Can you work these out from the model? Positions are in its coordinate system, mm. Round coordinates to 2 decimals unless told otherwise and drop trailing zeros.
Q1. Please list where these lines run through material, in increasing order: line 1 along Y through (x, z) = (-75, 12.5); line 2 along Y through (x, z) = (0, 32); line 3 along X through (y, z) = (46.5, 26).
Q2. We'd pull the mould along Y, two halves only. Please class faces 1 (the cylindrical face through (-19.527, 148.724, 39.44)), 2 (the cylindrical face through (-4.357, 54.908, 39.44)), 3 (the flat face through (32, -1, 80)), 4 (the cylindrical face through (23.1, 125.81, 39.44)): +Y half, -Y half, draft (parallel to the pull), parting line (faces both ways), or undercut.
Q3. If we section it at A-A (y = 0): Give the number of separate pieces and of enclosed holes in the cut face, plus the area to 3 significant figures.
Q4. I'm going to push flat-ended pins straight in: pin 1 Ø2 at (y, z) = (-83, 17.5) entering from -X; pin 2 Ø1.5 at (y, z) = (12.5, 24.5) entering from +X; pin 3 Ø8 at (y, z) = (17, 11.5) entering from +X. Where does each tip first touch, or does it pass through?
from build123d import *

# Parameters (mm, degrees)
SKETCH1_R           = 150
BOSS_EXTRUDE1_DEPTH = 80
BOSS_EXTRUDE2_DEPTH = 80
LOFT1_DEPTH         = 80
CIRPATTERN1_COUNT   = 5
FILLET1_R           = 20
FILLET2_R           = 20
FILLET3_R           = 20
SKETCH3_R           = 25
CUT_EXTRUDE1_DEPTH  = 80


with BuildPart() as part:
    # Sketch1 → Boss-Extrude1 (new body)
    with BuildSketch(Plane.XY):
        Circle(SKETCH1_R)
        with BuildLine():
            Line((129.710171657, 8.675907367), (119.956691368, 8.625091073))
            Line((119.956691368, 8.625091073), (120.040051321, -7.374691773))
            Line((120.040051321, -7.374691773), (129.793531611, -7.323875479))
            ThreePointArc((129.793531611, -7.323875479), (105.568888587, -75.86309882), (48.333925621, -120.680701166))
            Line((48.333925621, -120.680701166), (45.271605291, -111.420293279))
            Line((45.271605291, -111.420293279), (30.080667198, -116.443778112))
            Line((30.080667198, -116.443778112), (33.142987529, -125.704185999))
            ThreePointArc((33.142987529, -125.704185999), (-39.527513828, -123.84496619), (-99.838162814, -83.260682474))
            Line((-99.838162814, -83.260682474), (-91.977300573, -77.486619356))
            Line((-91.977300573, -77.486619356), (-101.449176589, -64.591520879))
            Line((-101.449176589, -64.591520879), (-109.310038829, -70.365583996))
            ThreePointArc((-109.310038829, -70.365583996), (-129.998235624, -0.677299621), (-110.037303615, 69.222769471))
            Line((-110.037303615, 69.222769471), (-102.116703238, 63.530928844))
            Line((-102.116703238, 63.530928844), (-92.779706461, 76.524022824))
            Line((-92.779706461, 76.524022824), (-100.700306837, 82.215863451))
            ThreePointArc((-100.700306837, 82.215863451), (-40.815814265, 123.426372003), (31.831369149, 126.042706802))
            Line((31.831369149, 126.042706802), (28.865707153, 116.750892719))
            Line((28.865707153, 116.750892719), (44.10816453, 111.88596794))
            Line((44.10816453, 111.88596794), (47.073826527, 121.177782024))
            ThreePointArc((47.073826527, 121.177782024), (104.772675129, 76.958992627), (129.710171657, 8.675907367))
        make_face(mode=Mode.SUBTRACT)
    extrude(amount=BOSS_EXTRUDE1_DEPTH)


with BuildPart() as body_2:
    # Sketch2 → Boss-Extrude2 (new body)
    with BuildSketch(Plane.XY):
        with BuildLine():
            Line((-5, 55), (5, 55))
            Line((5, 55), (5, 49.749371855))
            ThreePointArc((5, 49.749371855), (29.389262615, 40.450849719), (45.769379313, 20.128683944))
            Line((45.769379313, 20.128683944), (50.763023424, 21.751217272))
            Line((50.763023424, 21.751217272), (53.853193368, 12.240652109))
            Line((53.853193368, 12.240652109), (48.859549256, 10.618118781))
            ThreePointArc((48.859549256, 10.618118781), (47.552825815, -15.450849719), (33.287032059, -37.309161029))
            Line((33.287032059, -37.309161029), (36.373273848, -41.557008429))
            Line((36.373273848, -41.557008429), (28.283103904, -47.434860952))
            Line((28.283103904, -47.434860952), (25.196862116, -43.187013552))
            ThreePointArc((25.196862116, -43.187013552), (0, -50), (-25.196862116, -43.187013552))
            Line((-25.196862116, -43.187013552), (-28.283103904, -47.434860952))
            Line((-28.283103904, -47.434860952), (-36.373273848, -41.557008429))
            Line((-36.373273848, -41.557008429), (-33.287032059, -37.309161029))
            ThreePointArc((-33.287032059, -37.309161029), (-47.552825815, -15.450849719), (-48.859549256, 10.618118781))
            Line((-48.859549256, 10.618118781), (-53.853193368, 12.240652109))
            Line((-53.853193368, 12.240652109), (-50.763023424, 21.751217272))
            Line((-50.763023424, 21.751217272), (-45.769379313, 20.128683944))
            ThreePointArc((-45.769379313, 20.128683944), (-29.389262615, 40.450849719), (-5, 49.749371855))
            Line((-5, 49.749371855), (-5, 55))
        make_face()
    extrude(amount=BOSS_EXTRUDE2_DEPTH)


with BuildPart() as body_3:
    # Loft1: read off the stored shape, not the designer's step
    # Loft1 outline → Loft1 (new body)
    with BuildSketch(Plane.XY):
        Polygon((44.10816453, 111.88596794), (28.865707153, 116.750892719), (-5, 55), (5, 55), align=None)
    extrude(amount=LOFT1_DEPTH)


with BuildPart() as cirpattern1_1:
    # CirPattern1: pattern copy
    add(body_3.part.rotate(Axis((0, 0, 0), (0, 0, 1)), 1 * 360 / CIRPATTERN1_COUNT))


with BuildPart() as cirpattern1_2:
    # CirPattern1: pattern copy
    add(body_3.part.rotate(Axis((0, 0, 0), (0, 0, 1)), 2 * 360 / CIRPATTERN1_COUNT))


with BuildPart() as cirpattern1_3:
    # CirPattern1: pattern copy
    add(body_3.part.rotate(Axis((0, 0, 0), (0, 0, 1)), 3 * 360 / CIRPATTERN1_COUNT))


with BuildPart() as cirpattern1_4:
    # CirPattern1: pattern copy
    add(body_3.part.rotate(Axis((0, 0, 0), (0, 0, 1)), 4 * 360 / CIRPATTERN1_COUNT))

    # Combine1: union body 2, part, body 3, CirPattern1_1, CirPattern1_2, CirPattern1_3
    add(body_2.part)
    add(part.part)
    add(body_3.part)
    add(cirpattern1_1.part)
    add(cirpattern1_2.part)
    add(cirpattern1_3.part)

    # Fillet1
    # the kernel refuses this fillet: 20 mm, written as the material it adds along each edge
    with BuildSketch(Plane(origin=(-91.977300573, -77.486619356, 0), x_dir=(-0.8059436548419507, -0.5919922509796886, 0), z_dir=(0, 0, 1)), Plane(origin=(45.271605291, -111.420293279, 0), x_dir=(0.31396780203564834, -0.9494336307951725, 0), z_dir=(0, 0, 1)), Plane(origin=(-102.116703238, 63.530928844, 0), x_dir=(-0.8120683737452884, 0.5835622986131666, 0), z_dir=(0, 0, 1))) as fillet1_piece_1:
        with BuildLine():
            CenterArc((FILLET1_R * 0.0966409957188, FILLET1_R), FILLET1_R, 258.96004162, 11.03995838)
            Line((-FILLET1_R * 0.0948525451909, FILLET1_R * 0.0185061264634), (0, 0))
            Line((0, 0), (FILLET1_R * 0.0966409957188, 0))
        make_face()
    extrude(amount=80)
    with BuildSketch(Plane(origin=(119.956691369, 8.625091073, 0), x_dir=(-0.9824782333673042, 0.1863773617139722, 0), z_dir=(0, 0, 1))) as fillet1_piece_2:
        with BuildLine():
            CenterArc((FILLET1_R * 0.0966409957054, -FILLET1_R), FILLET1_R, 90, 11.03995838)
            Line((-FILLET1_R * 0.0948525452044, -FILLET1_R * 0.0185061264634), (0, 0))
            Line((0, 0), (FILLET1_R * 0.0966409957054, 0))
        make_face()
    extrude(amount=80)
    with BuildSketch(Plane(origin=(28.865707153, 116.750892719, 0), x_dir=(-0.4808578750966385, -0.8767985538067142, 0), z_dir=(0, 0, 1))) as fillet1_piece_3:
        with BuildLine():
            CenterArc((FILLET1_R * 0.0966409957188, -FILLET1_R), FILLET1_R, 90.000000002, 11.03995838)
            Line((-FILLET1_R * 0.0948525452298, -FILLET1_R * 0.018506126471), (0, 0))
            Line((0, 0), (FILLET1_R * 0.0966409956792, 0))
        make_face()
    extrude(amount=80)
    with BuildSketch(Plane(origin=(-36.373273848, -41.557008429, 0), x_dir=(-0.9426873980194184, -0.33367719372977617, 0), z_dir=(0, 0, 1)), Plane(origin=(28.283103904, -47.434860952, 0), x_dir=(0.026039443064681988, -0.9996609162135335, 0), z_dir=(0, 0, 1)), Plane(origin=(53.853193368, 12.240652109, 0), x_dir=(0.9587806588816111, -0.28414722971470946, 0), z_dir=(0, 0, 1)), Plane(origin=(5, 55, 0), x_dir=(0.5665195918801321, 0.8240482704404934, 0), z_dir=(0, 0, 1)), Plane(origin=(-50.763023424, 21.751217272, 0), x_dir=(-0.6086522958068845, 0.7934370692178484, 0), z_dir=(0, 0, 1))) as fillet1_piece_4:
        with BuildLine():
            CenterArc((6.167760881, -20), FILLET1_R, 90, 31.649839664)
            Line((-4.326771041, -2.974583714), (0, 0))
            Line((0, 0), (6.167760881, 0))
        make_face()
    extrude(amount=80)
    # the kernel refuses this fillet: 20 mm, written as the material it takes off along each edge
    with BuildSketch(Plane(origin=(-101.449176589, -64.591520879, -7.386208111), x_dir=(0.9426873980435565, 0.33367719366158266, 0), z_dir=(0, 0, 1)), Plane(origin=(30.080667198, -116.443778112, -7.386208111), x_dir=(-0.026039442992376174, 0.9996609162154169, 0), z_dir=(0, 0, 1)), Plane(origin=(44.10816453, 111.88596794, -7.386208111), x_dir=(-0.566519591939725, -0.8240482703995243, 0), z_dir=(0, 0, 1)), Plane(origin=(-92.779706461, 76.524022824, -7.386208111), x_dir=(0.6086522957494933, -0.7934370692618736, 0), z_dir=(0, 0, 1))) as fillet1_2_piece_1:
        with BuildLine():
            CenterArc((FILLET1_R * 0.147724162219, -FILLET1_R), FILLET1_R, 90.000000004, 16.806393351)
            Line((-FILLET1_R * 0.141414455522, -FILLET1_R * 0.042712760071), (0, 0))
            Line((0, 0), (FILLET1_R * 0.147724162147, 0))
        make_face()
    extrude(amount=94.772416222, mode=Mode.SUBTRACT)
    with BuildSketch(Plane(origin=(120.040051322, -7.374691773, -7.38620811), x_dir=(-0.9587806588816119, 0.2841472297147065, 0), z_dir=(0, 0, 1))) as fillet1_2_piece_2:
        with BuildLine():
            CenterArc((FILLET1_R * 0.14772416216, -FILLET1_R), FILLET1_R, 90, 16.806393351)
            Line((-FILLET1_R * 0.141414455511, -FILLET1_R * 0.04271276005), (0, 0))
            Line((0, 0), (FILLET1_R * 0.14772416216, 0))
        make_face()
    extrude(amount=94.77241622, mode=Mode.SUBTRACT)
    with BuildSketch(Plane(origin=(-28.283103904, -47.434860952, -12.810588384), x_dir=(-0.9043914519746539, -0.426703763277496, 0), z_dir=(0, 0, 1)), Plane(origin=(36.373273848, -41.557008429, -12.810588384), x_dir=(0.12634706636512016, -0.9919860980986216, 0), z_dir=(0, 0, 1)), Plane(origin=(50.763023424, 21.751217272, -12.810588384), x_dir=(0.9824782333673043, -0.18637736171397165, 0), z_dir=(0, 0, 1)), Plane(origin=(-53.853193368, 12.240652109, -12.810588384), x_dir=(-0.6852917228203294, 0.7282686692656392, 0), z_dir=(0, 0, 1))) as fillet1_2_piece_3:
        with BuildLine():
            CenterArc((FILLET1_R * 0.256211767685, -FILLET1_R), FILLET1_R, 90, 28.741446185)
            Line((-FILLET1_R * 0.224646107378, -FILLET1_R * 0.123201446175), (0, 0))
            Line((0, 0), (FILLET1_R * 0.256211767684, 0))
        make_face()
    extrude(amount=105.621176768, mode=Mode.SUBTRACT)
    with BuildSketch(Plane(origin=(-5, 55, -12.810588384), x_dir=(0, -1, 0), z_dir=(0, 0, 1))) as fillet1_2_piece_4:
        with BuildLine():
            CenterArc((FILLET1_R * 0.256211767684, FILLET1_R), FILLET1_R, 241.258553815, 28.741446185)
            Line((-FILLET1_R * 0.224646107378, FILLET1_R * 0.123201446174), (0, 0))
            Line((0, 0), (FILLET1_R * 0.256211767684, 0))
        make_face()
    extrude(amount=105.621176768, mode=Mode.SUBTRACT)

    # Fillet2
    fillet2_edges = [cirpattern1_4.edges().sort_by_distance(p)[0] for p in [
        (-45.769379313, 20.128683944, 40),
        (5, 49.749371855, 40),
        (48.859549256, 10.618118781, 40),
        (25.196862116, -43.187013552, 40),
        (-33.287032059, -37.309161029, 40),
    ]]
    fillet(fillet2_edges, radius=FILLET2_R - 0.0001)  # a hair under: the kernel refuses the full size

    # Fillet3
    # the kernel refuses this fillet: 20 mm, written as the material it adds along each edge
    with BuildSketch(Plane(origin=(-99.838162814, -83.260682474, 0), x_dir=(0.6928923413155604, -0.7210410552432093, 0), z_dir=(0, 0, 1)), Plane(origin=(48.333925621, -120.680701166, 0), x_dir=(0.899866302844142, 0.43616583658697394, 0), z_dir=(0, 0, 1)), Plane(origin=(129.710171657, 8.675907367, 0), x_dir=(-0.1367443808271708, 0.9906063669854912, 0), z_dir=(0, 0, 1)), Plane(origin=(31.831369149, 126.042706802, 0), x_dir=(-0.9843789779658949, 0.17606256768211787, 0), z_dir=(0, 0, 1)), Plane(origin=(-110.037303615, 69.222769471, 0), x_dir=(-0.4716352853666361, -0.881793716011365, 0), z_dir=(0, 0, 1))) as fillet3_piece_1:
        with BuildLine():
            CenterArc((16.878882523, 19.95047746), FILLET3_R, 217.581129198, 56.451736362)
            Line((1.029071396, 7.752793776), (0.712075174, 7.508840102))
            ThreePointArc((0.712075174, 7.508840102), (0.118013554, 3.929029475), (-0.396522144, 0.052632587))
            Line((-0.396522144, 0.052632587), (-0.028131471, -0.399009549))
            ThreePointArc((-0.028131471, -0.399009549), (9.142728033, -0.721896513), (18.313587537, -0.399009549))
            Line((18.313587537, -0.399009549), (18.285456067, 0))
        make_face()
    extrude(amount=80)

    # Sketch3 → Cut-Extrude1 (cut)
    with BuildSketch(Plane.XY.offset(80)):
        Circle(SKETCH3_R)
    extrude(amount=-CUT_EXTRUDE1_DEPTH, mode=Mode.SUBTRACT)


solid = cirpattern1_4.part
A:
1. line 1: y = -129.9 to -106.18, -69.48 to -55.23, 34.71 to 53.35, 106.18 to 129.9
1. line 2: y = -150 to -130, -50 to -25, 25 to 64.12, 130 to 150
1. line 3: x = -142.61 to -121.4, -86.09 to -69.75, -18.38 to 20.29, 121.4 to 142.61
2. face 1: parting line
2. face 2: undercut
2. face 3: draft
2. face 4: undercut
3. separate pieces: 4
3. enclosed holes: 0
3. area: 10,300 mm2
4. pin 1: stops at x = -125.6
4. pin 2: stops at x = 149.54
4. pin 3: stops at x = 149.44
